For this review, use the dimensioned drawing (mm, ordinates from the lowest corner) and the shaded views. Coordinates: 2 decimals unless noted, no trailing zeros. Write each loop counter-clockwise with the first axis right and the second up, starting at its lowest first coordinate (ties: lowest second). Pieces come first, ordered by that corner, then holes.
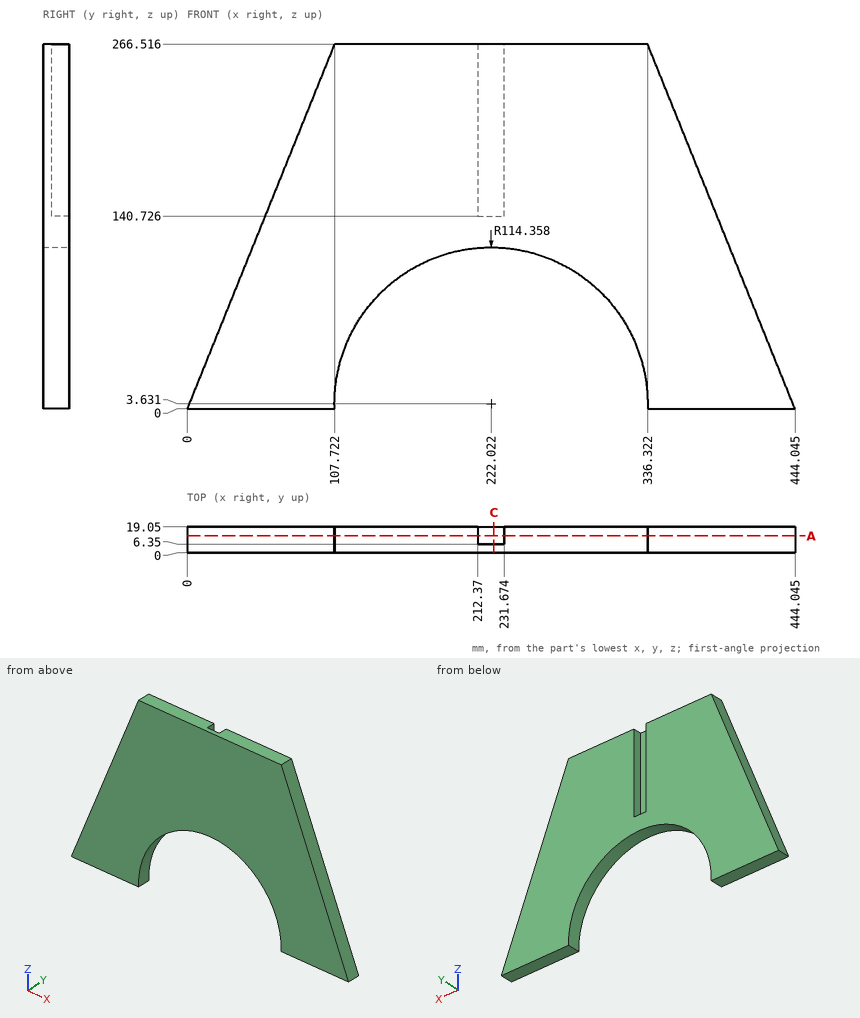
Item 1: Take a section at A-A, the plane y = 12.5. Write out the cut boundary in (x, z) (1 decimal).
Solved:
outline: (0, 0) - (107.7, 0) arc R114.4 cw (long way) to (336.3, 0) - (444, 0) - (336.3, 266.5) - (231.7, 266.5) - (231.7, 140.7) - (212.4, 140.7) - (212.4, 266.5) - (107.7, 266.5) - close
Item 2: To check wall thickness, follow line 1 along X through (y, z) = (11, 36.5) (1 decimal); line 2 along X through (y, z) = (18.25, 186) (1 decimal); line 3 along Z through (x, y) = (269, 11.75) (1 decimal). State the ranges of each line that lie inside material, in increasing order.
Solved:
line 1: x = 14.8 to 112.5, 331.6 to 429.3
line 2: x = 75.2 to 212.4, 231.7 to 368.9
line 3: z = 107.9 to 266.5
Item 3: Take a section at C-C, the plane x = 224. Write out the cut boundary in (y, z).
Solved:
outline: (0, 117.97) - (19.05, 117.97) - (19.05, 140.73) - (6.35, 140.73) - (6.35, 266.52) - (0, 266.52) - close
Item 4: For pin 1 (10 mm diameter, centred on y = 12.5, z = 212, fed in from -X); pin 2 (5 mm diameter, centred on y = 9, z = 70, fed in from +X); pin 3 (6.5 mm diameter, centred on x = 217.5, y = 15.5, fed in from +Z), all flat-tipped, find the tip position at first contact; note any pin that passes through.
Solved:
pin 1: stops at x = 83.67
pin 2: stops at x = 416.76
pin 3: stops at z = 140.73
